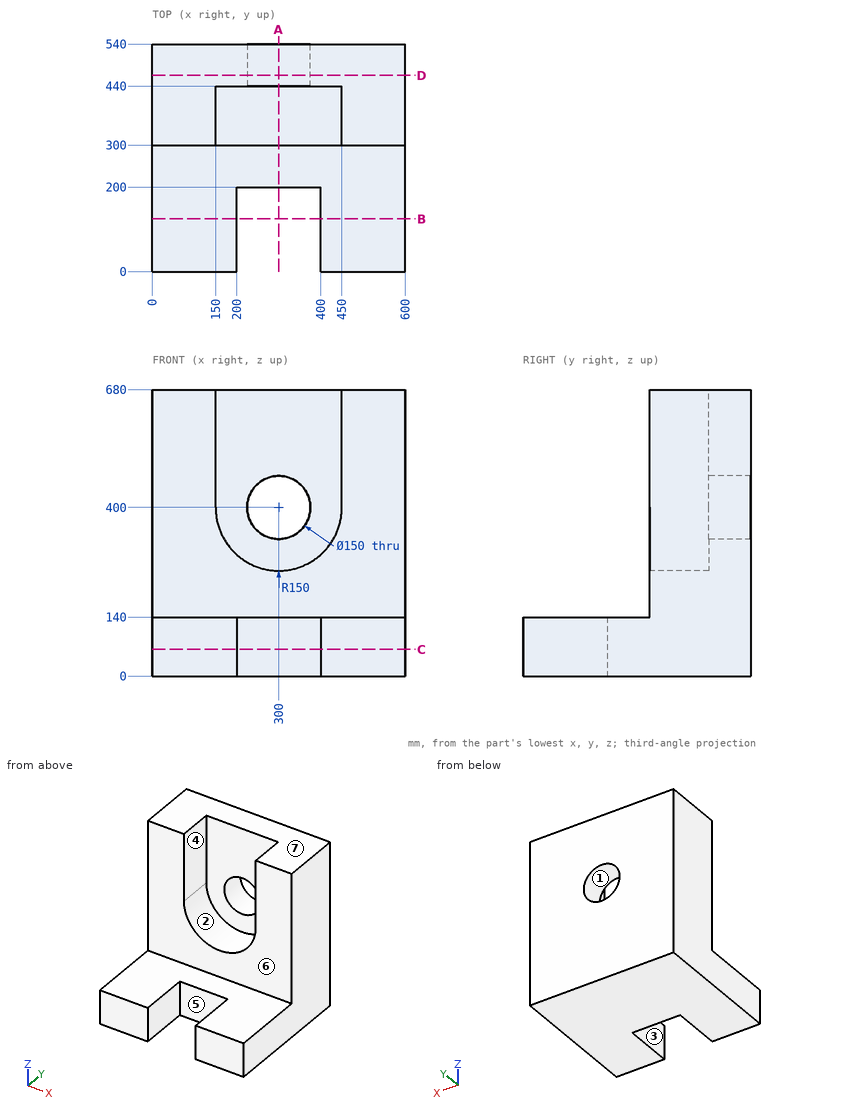
Input: dimensioned drawing with shaded views. Units: mm. Origin: part minimum x, y, z. A direction names the side the tool comes from. Coordinates: 2 decimals unless noted, no trailing zeros. Loops run counter-clockwise (first coordinate to the right, second up) from the corner with the lowest first, then second, coordinate; pieces in that order, holes last. Notation, with made-up numbers: (55, -23) -> (110, -23) arc R26 ccw to (110, 4) -> close; hole circle Ø11 at (-24.75, 73). An arc over 180 degrees is marked (long way). Use a Markdown table: item, result. Add a question column.
(1) Line query: line 1 along X through (y, z) = (318.5, 421); line 2 along Z through (x, y) = (300, 476); line 3 along Y through (x, z) = (111.5, 248.5). Output: solid intervals per line, ascending.
(2) Section query D-D, the plane y = 465.5. Return loops of the section in (x, z), plus the area to 3 significant figures.
(3) Section query C-C, the plane z = 63. Return loops of the section in (x, y), plus the area to 3 significant figures.
(4) Pin query (flat end, axial travel): pin 1 Ø6 at (x, z) = (195, 430) entering from -Y; pin 2 Ø4 at (x, y) = (190.5, 152.5) entering from +Z. Return the tip coordinate at first contact, or that it passes through.
(5) Section query B-B, the plane y = 125. Return loops of the section in (x, z).
(6) Mould query, pull axis Z, two halves, no side actions, for the marked faces 1, 2 and 3. Classes: pulls with the +Z half, pulls with the -Z half, needs draft (parallel to the pull), parting line crosses it, or undercut.
(7) Section query A-A, the plane x = 300. Return loops of the section in (y, z).
(8) Access query for the marked faces 4, 5, 6 and 7. Directions: +Z, -Z, +X, -X, +Y, -Y. A direction counts if a zero-diameter tool reaches every point of the face in a straight line with its end or side. Return the directions, or none.
Answer:
| question | item | result |
|---|---|---|
| 1 | line 1 | x = 0 to 150, 450 to 600 |
| 1 | line 2 | z = 0 to 325, 475 to 680 |
| 1 | line 3 | y = 300 to 540 |
| 2 | outline | (0, 0) -> (600, 0) -> (600, 680) -> (0, 680) -> close; hole circle Ø150 at (300, 400) |
| 2 | area | 390,000 mm^2 |
| 3 | outline | (0, 0) -> (200, 0) -> (200, 200) -> (400, 200) -> (400, 0) -> (600, 0) -> (600, 540) -> (0, 540) -> close |
| 3 | area | 284,000 mm^2 |
| 4 | pin 1 | stops at y = 440 |
| 4 | pin 2 | stops at z = 140 |
| 5 | outline | (0, 0) -> (200, 0) -> (200, 140) -> (0, 140) -> close; (400, 0) -> (600, 0) -> (600, 140) -> (400, 140) -> close |
| 6 | face 1 | undercut |
| 6 | face 2 | pulls with the +Z half |
| 6 | face 3 | needs draft |
| 7 | outline | (200, 0) -> (540, 0) -> (540, 325) -> (440, 325) -> (440, 250) -> (300, 250) -> (300, 140) -> (200, 140) -> close; (440, 475) -> (540, 475) -> (540, 680) -> (440, 680) -> close |
| 8 | face 4 | +Z, -Y |
| 8 | face 5 | +Z, -Z, -Y |
| 8 | face 6 | +Z, +X, -X, -Y |
| 8 | face 7 | +Z, +X, -X, +Y, -Y |
